Could you check a few things on this model? Use its own coordinates, in mm. A direction names the side the tool comes from. Coordinates: 2 decimals unless noted, no trailing zeros. Order: outer loops, then holes, each group sorted by start corner. A loop starts at its lowest first (then second) coordinate and runs counter-clockwise, first axis right, second up.
```python
from build123d import *

# Parameters (mm, degrees)
ESBO_O1_W                = 99.1
ESBO_O1_H                = 166.52
RESSALTO_EXTRUS_O1_DEPTH = 5
FILETE1_R                = 3
ESBO_O2_R                = 3.1
CORTE_EXTRUS_O1_DEPTH    = 1.6
ESBO_O3_R                = 3.1
CORTE_EXTRUS_O2_DEPTH    = 1.6
ESBO_O4_R                = 3.1
CORTE_EXTRUS_O3_DEPTH    = 1.6
ESBO_O5_R                = 3.1
CORTE_EXTRUS_O4_DEPTH    = 1.6
ESBO_O6_R                = 7
CORTE_EXTRUS_O5_DEPTH    = 10


with BuildPart() as part:
    # Esboço1 → Ressalto-extrusão1 (new body)
    with BuildSketch(Plane.XY):
        with Locations((5.497464185, 11.397762804)):
            Rectangle(ESBO_O1_W, ESBO_O1_H)
    extrude(amount=RESSALTO_EXTRUS_O1_DEPTH)

    # Filete1
    filete1_edges = [part.edges().sort_by_distance(p)[0] for p in [
        (55.047464185, 11.397762804, 5),
        (5.497464185, 94.657762804, 5),
        (-44.052535815, 11.397762804, 5),
        (5.497464185, -71.862237196, 5),
    ]]
    fillet(filete1_edges, radius=FILETE1_R)

    # Esboço2 → Corte-extrusão1 (cut)
    with BuildSketch(Plane(origin=(0, 0, 0), x_dir=(-1, 0, 0), z_dir=(0, 0, -1))):
        with Locations((-51.497464185, 91.107762804)):
            Circle(ESBO_O2_R)
    extrude(amount=-CORTE_EXTRUS_O1_DEPTH, mode=Mode.SUBTRACT)

    # Esboço3 → Corte-extrusão2 (cut)
    with BuildSketch(Plane(origin=(0, 0, 0), x_dir=(-1, 0, 0), z_dir=(0, 0, -1))):
        with Locations((40.502535815, 91.107762804)):
            Circle(ESBO_O3_R)
    extrude(amount=-CORTE_EXTRUS_O2_DEPTH, mode=Mode.SUBTRACT)

    # Esboço4 → Corte-extrusão3 (cut)
    with BuildSketch(Plane(origin=(0, 0, 0), x_dir=(-1, 0, 0), z_dir=(0, 0, -1))):
        with Locations((-51.497464185, -68.312237196)):
            Circle(ESBO_O4_R)
    extrude(amount=-CORTE_EXTRUS_O3_DEPTH, mode=Mode.SUBTRACT)

    # Esboço5 → Corte-extrusão4 (cut)
    with BuildSketch(Plane(origin=(0, 0, 0), x_dir=(-1, 0, 0), z_dir=(0, 0, -1))):
        with Locations((40.502535815, -68.312237196)):
            Circle(ESBO_O5_R)
    extrude(amount=-CORTE_EXTRUS_O4_DEPTH, mode=Mode.SUBTRACT)

    # Esboço6 → Corte-extrusão5 (cut)
    with BuildSketch(Plane(origin=(0, 0, 0), x_dir=(-1, 0, 0), z_dir=(0, 0, -1))):
        with Locations((-5.41867497, 83.857762804)):
            Circle(ESBO_O6_R)
    extrude(amount=-CORTE_EXTRUS_O5_DEPTH, mode=Mode.SUBTRACT)


solid = part.part
```
Item 1: Thinking about a two-plate mould opening in X: for faces 1 (the face through (6.2, 93.8, 4.1)), 2 (the face through (54.19, 12.56, 4.1)), 3 (the face through (-38.218, 93.203, 0.789)), which applies, +X half, -X half, draft (parallel to the pull), parting line (faces both ways), or undercut?
Item 2: Which directions (+Z, -Z, +X, -X, +Y, -Y) give clear straight access to the entire face, cutting with the end or side of a thin tool? Please do faces 4 (the face through (6.191, -71.007, 4.098)), 5 (the face through (53.782, 93.203, 0.789)).
Item 3: I need wall thicknesses on line 1 (Y direction, x = -0.5, z = 3.25); line 2 (X direction, y = -15, z = 2.4); line 3 (Y direction, x = -0.5, z = 3). Which ranges of each line are inside material? Lowest first, please.
Item 4: For pin 1 Ø1.9 at (x, y) = (-39.5, 92.5) entering from -Z, with a flat end and sliding along its axis, tell me the tip position at first contact or that it passes through.
Item 5: Suppose I cut it at A-A (z = 4). List the corners of the cut face in (x, y) for me.
Geometry results:
1. face 1: draft
1. face 2: +X half
1. face 3: undercut
2. face 4: +Z, +X, -X, -Y
2. face 5: -Z
3. line 1: y = -71.59 to 80.12, 87.6 to 94.38
3. line 2: x = -44.03 to 55.02
3. line 3: y = -71.69 to 80.12, 87.6 to 94.49
4. pin 1: stops at z = 1.6
5. outline: (-43.29, -71.1) - (54.28, -71.1) - (54.28, 93.89) - (-43.29, 93.89) - close; hole circle Ø14 at (5.42, 83.86)
